Source: CAD feature listing. Evaluate the final solid. Frame: model axes, mm. A direction names the side the tool comes from. Give positions to 0.01 mm unless a question says otherwise; leave off trailing zeros. Order: outer loops, then holes, each group sorted by start corner. A loop starts at its lowest first (then second) coordinate and runs counter-clockwise, first axis right, second up.
```python
from build123d import *

# Parameters (mm, degrees)
BOX029_W     = 6
BOX029_H     = 13
BOX029_DEPTH = 18
BOX027_W     = 4
BOX027_H     = 1.25
BOX027_DEPTH = 3
BOX026_W     = 4
BOX026_H     = 1.25
BOX026_DEPTH = 3
BOX028_W     = 4
BOX028_H     = 1.25
BOX028_DEPTH = 3
BOX025_W     = 4
BOX025_H     = 4
BOX025_DEPTH = 1.25
BOX024_W     = 4
BOX024_H     = 4
BOX024_DEPTH = 1.25
BOX023_W     = 4
BOX023_H     = 4
BOX023_DEPTH = 1.25
BOX022_W     = 4
BOX022_H     = 4
BOX022_DEPTH = 1.25
BOX021_W     = 4
BOX021_H     = 4
BOX021_DEPTH = 1.25
BOX020_W     = 4
BOX020_H     = 4
BOX020_DEPTH = 1.25
BOX019_W     = 4
BOX019_H     = 4
BOX019_DEPTH = 1.25
BOX018_W     = 4
BOX018_H     = 4
BOX018_DEPTH = 1.25
BOX017_W     = 4
BOX017_H     = 4
BOX017_DEPTH = 1.25
BOX016_W     = 4
BOX016_H     = 4
BOX016_DEPTH = 1.25
BOX015_W     = 7
BOX015_H     = 1.25
BOX015_DEPTH = 1.25
BOX014_W     = 7
BOX014_H     = 1.25
BOX014_DEPTH = 1.25
BOX013_W     = 7
BOX013_H     = 1.25
BOX013_DEPTH = 1.25
BOX012_W     = 7
BOX012_H     = 1.25
BOX012_DEPTH = 1.25
BOX011_W     = 7
BOX011_H     = 1.25
BOX011_DEPTH = 1.25
BOX010_W     = 7
BOX010_H     = 1.25
BOX010_DEPTH = 1.25
BOX009_W     = 7
BOX009_H     = 1.25
BOX009_DEPTH = 1.25
BOX008_W     = 7
BOX008_H     = 1.25
BOX008_DEPTH = 1.25
BOX007_W     = 7
BOX007_H     = 1.25
BOX007_DEPTH = 1.25
BOX006_W     = 7
BOX006_H     = 1.25
BOX006_DEPTH = 1.25
BOX005_W     = 7
BOX005_H     = 1.25
BOX005_DEPTH = 1.25
BOX004_W     = 7
BOX004_H     = 1.25
BOX004_DEPTH = 1.25
BOX003_W     = 7
BOX003_H     = 1.25
BOX003_DEPTH = 1.25
BOX002_W     = 7
BOX002_H     = 1.25
BOX002_DEPTH = 1.25
BOX001_W     = 7
BOX001_H     = 1.25
BOX001_DEPTH = 1.25
BOX_W        = 8
BOX_H        = 15
BOX_DEPTH    = 20


with BuildPart() as middle:
    # Box029 → Box029 (new body)
    with BuildSketch(Plane(origin=(1, 1, 2), x_dir=(1, 0, 0), z_dir=(0, 0, 1))):
        with Locations((3, 6.5)):
            Rectangle(BOX029_W, BOX029_H)
    extrude(amount=BOX029_DEPTH)


with BuildPart() as cube027:
    # Box027 → Box027 (new body)
    with BuildSketch(Plane(origin=(4, 7, 18), x_dir=(1, 0, 0), z_dir=(0, 0, 1))):
        with Locations((2, 0.625)):
            Rectangle(BOX027_W, BOX027_H)
    extrude(amount=BOX027_DEPTH)


with BuildPart() as cube026:
    # Box026 → Box026 (new body)
    with BuildSketch(Plane(origin=(4, 9, 18), x_dir=(1, 0, 0), z_dir=(0, 0, 1))):
        with Locations((2, 0.625)):
            Rectangle(BOX026_W, BOX026_H)
    extrude(amount=BOX026_DEPTH)


with BuildPart() as cube028:
    # Box028 → Box028 (new body)
    with BuildSketch(Plane(origin=(4, 5, 18), x_dir=(1, 0, 0), z_dir=(0, 0, 1))):
        with Locations((2, 0.625)):
            Rectangle(BOX028_W, BOX028_H)
    extrude(amount=BOX028_DEPTH)


with BuildPart() as cube025:
    # Box025 → Box025 (new body)
    with BuildSketch(Plane(origin=(4, 11, 5), x_dir=(1, 0, 0), z_dir=(0, 0, 1))):
        with Locations((2, 2)):
            Rectangle(BOX025_W, BOX025_H)
    extrude(amount=BOX025_DEPTH)


with BuildPart() as cube024:
    # Box024 → Box024 (new body)
    with BuildSketch(Plane(origin=(4, 11, 7.5), x_dir=(1, 0, 0), z_dir=(0, 0, 1))):
        with Locations((2, 2)):
            Rectangle(BOX024_W, BOX024_H)
    extrude(amount=BOX024_DEPTH)


with BuildPart() as cube023:
    # Box023 → Box023 (new body)
    with BuildSketch(Plane(origin=(4, 11, 10), x_dir=(1, 0, 0), z_dir=(0, 0, 1))):
        with Locations((2, 2)):
            Rectangle(BOX023_W, BOX023_H)
    extrude(amount=BOX023_DEPTH)


with BuildPart() as cube022:
    # Box022 → Box022 (new body)
    with BuildSketch(Plane(origin=(4, 11, 12.5), x_dir=(1, 0, 0), z_dir=(0, 0, 1))):
        with Locations((2, 2)):
            Rectangle(BOX022_W, BOX022_H)
    extrude(amount=BOX022_DEPTH)


with BuildPart() as cube021:
    # Box021 → Box021 (new body)
    with BuildSketch(Plane(origin=(4, 11, 15), x_dir=(1, 0, 0), z_dir=(0, 0, 1))):
        with Locations((2, 2)):
            Rectangle(BOX021_W, BOX021_H)
    extrude(amount=BOX021_DEPTH)


with BuildPart() as cube020:
    # Box020 → Box020 (new body)
    with BuildSketch(Plane(origin=(4, 0, 15), x_dir=(1, 0, 0), z_dir=(0, 0, 1))):
        with Locations((2, 2)):
            Rectangle(BOX020_W, BOX020_H)
    extrude(amount=BOX020_DEPTH)


with BuildPart() as cube019:
    # Box019 → Box019 (new body)
    with BuildSketch(Plane(origin=(4, 0, 12.5), x_dir=(1, 0, 0), z_dir=(0, 0, 1))):
        with Locations((2, 2)):
            Rectangle(BOX019_W, BOX019_H)
    extrude(amount=BOX019_DEPTH)


with BuildPart() as cube018:
    # Box018 → Box018 (new body)
    with BuildSketch(Plane(origin=(4, 0, 10), x_dir=(1, 0, 0), z_dir=(0, 0, 1))):
        with Locations((2, 2)):
            Rectangle(BOX018_W, BOX018_H)
    extrude(amount=BOX018_DEPTH)


with BuildPart() as cube017:
    # Box017 → Box017 (new body)
    with BuildSketch(Plane(origin=(4, 0, 7.5), x_dir=(1, 0, 0), z_dir=(0, 0, 1))):
        with Locations((2, 2)):
            Rectangle(BOX017_W, BOX017_H)
    extrude(amount=BOX017_DEPTH)


with BuildPart() as cube016:
    # Box016 → Box016 (new body)
    with BuildSketch(Plane(origin=(4, 0, 5), x_dir=(1, 0, 0), z_dir=(0, 0, 1))):
        with Locations((2, 2)):
            Rectangle(BOX016_W, BOX016_H)
    extrude(amount=BOX016_DEPTH)


with BuildPart() as cube015:
    # Box015 → Box015 (new body)
    with BuildSketch(Plane(origin=(1, 9, 5), x_dir=(1, 0, 0), z_dir=(0, 0, 1))):
        with Locations((3.5, 0.625)):
            Rectangle(BOX015_W, BOX015_H)
    extrude(amount=BOX015_DEPTH)


with BuildPart() as cube014:
    # Box014 → Box014 (new body)
    with BuildSketch(Plane(origin=(1, 7, 5), x_dir=(1, 0, 0), z_dir=(0, 0, 1))):
        with Locations((3.5, 0.625)):
            Rectangle(BOX014_W, BOX014_H)
    extrude(amount=BOX014_DEPTH)


with BuildPart() as cube013:
    # Box013 → Box013 (new body)
    with BuildSketch(Plane(origin=(1, 5, 5), x_dir=(1, 0, 0), z_dir=(0, 0, 1))):
        with Locations((3.5, 0.625)):
            Rectangle(BOX013_W, BOX013_H)
    extrude(amount=BOX013_DEPTH)


with BuildPart() as cube012:
    # Box012 → Box012 (new body)
    with BuildSketch(Plane(origin=(1, 5, 7.5), x_dir=(1, 0, 0), z_dir=(0, 0, 1))):
        with Locations((3.5, 0.625)):
            Rectangle(BOX012_W, BOX012_H)
    extrude(amount=BOX012_DEPTH)


with BuildPart() as cube011:
    # Box011 → Box011 (new body)
    with BuildSketch(Plane(origin=(1, 7, 7.5), x_dir=(1, 0, 0), z_dir=(0, 0, 1))):
        with Locations((3.5, 0.625)):
            Rectangle(BOX011_W, BOX011_H)
    extrude(amount=BOX011_DEPTH)


with BuildPart() as cube010:
    # Box010 → Box010 (new body)
    with BuildSketch(Plane(origin=(1, 7, 10), x_dir=(1, 0, 0), z_dir=(0, 0, 1))):
        with Locations((3.5, 0.625)):
            Rectangle(BOX010_W, BOX010_H)
    extrude(amount=BOX010_DEPTH)


with BuildPart() as cube009:
    # Box009 → Box009 (new body)
    with BuildSketch(Plane(origin=(1, 9, 7.5), x_dir=(1, 0, 0), z_dir=(0, 0, 1))):
        with Locations((3.5, 0.625)):
            Rectangle(BOX009_W, BOX009_H)
    extrude(amount=BOX009_DEPTH)


with BuildPart() as cube008:
    # Box008 → Box008 (new body)
    with BuildSketch(Plane(origin=(1, 9, 10), x_dir=(1, 0, 0), z_dir=(0, 0, 1))):
        with Locations((3.5, 0.625)):
            Rectangle(BOX008_W, BOX008_H)
    extrude(amount=BOX008_DEPTH)


with BuildPart() as cube007:
    # Box007 → Box007 (new body)
    with BuildSketch(Plane(origin=(1, 5, 10), x_dir=(1, 0, 0), z_dir=(0, 0, 1))):
        with Locations((3.5, 0.625)):
            Rectangle(BOX007_W, BOX007_H)
    extrude(amount=BOX007_DEPTH)


with BuildPart() as cube006:
    # Box006 → Box006 (new body)
    with BuildSketch(Plane(origin=(1, 5, 12.5), x_dir=(1, 0, 0), z_dir=(0, 0, 1))):
        with Locations((3.5, 0.625)):
            Rectangle(BOX006_W, BOX006_H)
    extrude(amount=BOX006_DEPTH)


with BuildPart() as cube005:
    # Box005 → Box005 (new body)
    with BuildSketch(Plane(origin=(1, 9, 12.5), x_dir=(1, 0, 0), z_dir=(0, 0, 1))):
        with Locations((3.5, 0.625)):
            Rectangle(BOX005_W, BOX005_H)
    extrude(amount=BOX005_DEPTH)


with BuildPart() as cube004:
    # Box004 → Box004 (new body)
    with BuildSketch(Plane(origin=(1, 7, 12.5), x_dir=(1, 0, 0), z_dir=(0, 0, 1))):
        with Locations((3.5, 0.625)):
            Rectangle(BOX004_W, BOX004_H)
    extrude(amount=BOX004_DEPTH)


with BuildPart() as cube003:
    # Box003 → Box003 (new body)
    with BuildSketch(Plane(origin=(1, 9, 15), x_dir=(1, 0, 0), z_dir=(0, 0, 1))):
        with Locations((3.5, 0.625)):
            Rectangle(BOX003_W, BOX003_H)
    extrude(amount=BOX003_DEPTH)


with BuildPart() as cube002:
    # Box002 → Box002 (new body)
    with BuildSketch(Plane(origin=(1, 7, 15), x_dir=(1, 0, 0), z_dir=(0, 0, 1))):
        with Locations((3.5, 0.625)):
            Rectangle(BOX002_W, BOX002_H)
    extrude(amount=BOX002_DEPTH)


with BuildPart() as cube001:
    # Box001 → Box001 (new body)
    with BuildSketch(Plane(origin=(1, 5, 15), x_dir=(1, 0, 0), z_dir=(0, 0, 1))):
        with Locations((3.5, 0.625)):
            Rectangle(BOX001_W, BOX001_H)
    extrude(amount=BOX001_DEPTH)


with BuildPart() as cut045:
    # Box → Box (new body)
    with BuildSketch(Plane.XY.offset(1)):
        with Locations((4, 7.5)):
            Rectangle(BOX_W, BOX_H)
    extrude(amount=BOX_DEPTH)

    # Cut: cut Cube001
    add(cube001.part, mode=Mode.SUBTRACT)

    # Cut001: cut Cube002
    add(cube002.part, mode=Mode.SUBTRACT)

    # Cut002: cut Cube003
    add(cube003.part, mode=Mode.SUBTRACT)

    # Cut003: cut Cube004
    add(cube004.part, mode=Mode.SUBTRACT)

    # Cut004: cut Cube005
    add(cube005.part, mode=Mode.SUBTRACT)

    # Cut005: cut Cube006
    add(cube006.part, mode=Mode.SUBTRACT)

    # Cut006: cut Cube007
    add(cube007.part, mode=Mode.SUBTRACT)

    # Cut007: cut Cube008
    add(cube008.part, mode=Mode.SUBTRACT)

    # Cut008: cut Cube009
    add(cube009.part, mode=Mode.SUBTRACT)

    # Cut009: cut Cube010
    add(cube010.part, mode=Mode.SUBTRACT)

    # Cut010: cut Cube011
    add(cube011.part, mode=Mode.SUBTRACT)

    # Cut011: cut Cube012
    add(cube012.part, mode=Mode.SUBTRACT)

    # Cut012: cut Cube013
    add(cube013.part, mode=Mode.SUBTRACT)

    # Cut013: cut Cube014
    add(cube014.part, mode=Mode.SUBTRACT)

    # Cut014: cut Cube015
    add(cube015.part, mode=Mode.SUBTRACT)

    # Cut032: cut Cube016
    add(cube016.part, mode=Mode.SUBTRACT)

    # Cut033: cut Cube017
    add(cube017.part, mode=Mode.SUBTRACT)

    # Cut034: cut Cube018
    add(cube018.part, mode=Mode.SUBTRACT)

    # Cut035: cut Cube019
    add(cube019.part, mode=Mode.SUBTRACT)

    # Cut036: cut Cube020
    add(cube020.part, mode=Mode.SUBTRACT)

    # Cut037: cut Cube021
    add(cube021.part, mode=Mode.SUBTRACT)

    # Cut038: cut Cube022
    add(cube022.part, mode=Mode.SUBTRACT)

    # Cut039: cut Cube023
    add(cube023.part, mode=Mode.SUBTRACT)

    # Cut040: cut Cube024
    add(cube024.part, mode=Mode.SUBTRACT)

    # Cut041: cut Cube025
    add(cube025.part, mode=Mode.SUBTRACT)

    # Cut042: cut Cube028
    add(cube028.part, mode=Mode.SUBTRACT)

    # Cut043: cut Cube026
    add(cube026.part, mode=Mode.SUBTRACT)

    # Cut044: cut Cube027
    add(cube027.part, mode=Mode.SUBTRACT)

    # Cut045: cut Middle
    add(middle.part, mode=Mode.SUBTRACT)


solid = cut045.part
```
1) Section query B-B, the plane x = 1.25. Return the cut outline in (y, z), and give its area (3 significant figures).
Report:
outline: (0, 1) - (15, 1) - (15, 21) - (0, 21) - close; hole (1, 2) - (14, 2) - (14, 20) - (1, 20) - close
area: 66.0 mm2
2) Reachability of faces 4 (the flat face through (7.5, 5.6, 16.25)), 5 (the flat face through (7.5, 11, 10.6)), 6 (the flat face through (7.5, 4, 15.6)), 7 (the flat face through (6.4, 7, 20.5)) from +Z, -Z, +X, -X, +Y, -Y: full face, straight path, thin tool, end or side. Return the list, or none.
Report:
face 4: +X
face 5: +X, +Y
face 6: +X, -Y
face 7: +Z, +X
3) Section query C-C, the plane y = 12. Return the cut outline in (x, z), and give its area (4 significant figures).
Report:
outline: (0, 1) - (8, 1) - (8, 5) - (7, 5) - (7, 2) - (1, 2) - (1, 20) - (7, 20) - (7, 16.25) - (8, 16.25) - (8, 21) - (0, 21) - close; (7, 6.25) - (8, 6.25) - (8, 7.5) - (7, 7.5) - close; (7, 8.75) - (8, 8.75) - (8, 10) - (7, 10) - close; (7, 11.25) - (8, 11.25) - (8, 12.5) - (7, 12.5) - close; (7, 13.75) - (8, 13.75) - (8, 15) - (7, 15) - close
area: 45.75 mm2
4) Section query A-A, the plane z = 5.25. Return the cut outline in (x, y).
Report:
outline: (0, 0) - (4, 0) - (4, 1) - (1, 1) - (1, 14) - (4, 14) - (4, 15) - (0, 15) - close; (7, 4) - (8, 4) - (8, 5) - (7, 5) - close; (7, 6.25) - (8, 6.25) - (8, 7) - (7, 7) - close; (7, 8.25) - (8, 8.25) - (8, 9) - (7, 9) - close; (7, 10.25) - (8, 10.25) - (8, 11) - (7, 11) - close
5) Section query D-D, the plane z = 19.25. Return the cut outline in (x, y).
Report:
outline: (0, 0) - (8, 0) - (8, 5) - (7, 5) - (7, 1) - (1, 1) - (1, 14) - (7, 14) - (7, 10.25) - (8, 10.25) - (8, 15) - (0, 15) - close; (7, 6.25) - (8, 6.25) - (8, 7) - (7, 7) - close; (7, 8.25) - (8, 8.25) - (8, 9) - (7, 9) - close
6) Pin query (flat end, axial travel): pin 1 (0.8 mm diameter, centred on x = 7.5, z = 15.5, fed in from -Y); pin 2 (0.5 mm diameter, centred on x = 7.5, z = 15.5, fed in from +Y); pin 3 (0.8 mm diameter, centred on y = 7.5, z = 20.5, fed in from +X). Return the tip coordinate at first contact, or that it passes through.
Report:
pin 1: stops at y = 4
pin 2: stops at y = 11
pin 3: stops at x = 4
7) Material intervals for L1, parallel to Z at x = 7.5, y = 1.25; L2, parallel to Z at x = 7.75, y = 6; L3, parallel to Y at x = 4.5, z = 20.25, sorted ascending.
Report:
L1: z = 1 to 5, 6.25 to 7.5, 8.75 to 10, 11.25 to 12.5, 13.75 to 15, 16.25 to 21
L2: z = 1 to 5, 6.25 to 7.5, 8.75 to 10, 11.25 to 12.5, 13.75 to 15, 16.25 to 18
L3: y = 0 to 5, 6.25 to 7, 8.25 to 9, 10.25 to 15
8) Draft query along X for faces 1 (the flat face through (3, 14, 11)), 2 (the flat face through (7.5, 6.25, 13.1)), 3 (the flat face through (4, 0.5, 10.6)). Return one class per face: +X half, -X half, draft (parallel to the pull), parting line (faces both ways), or undercut.
Report:
face 1: undercut
face 2: draft
face 3: +X half
